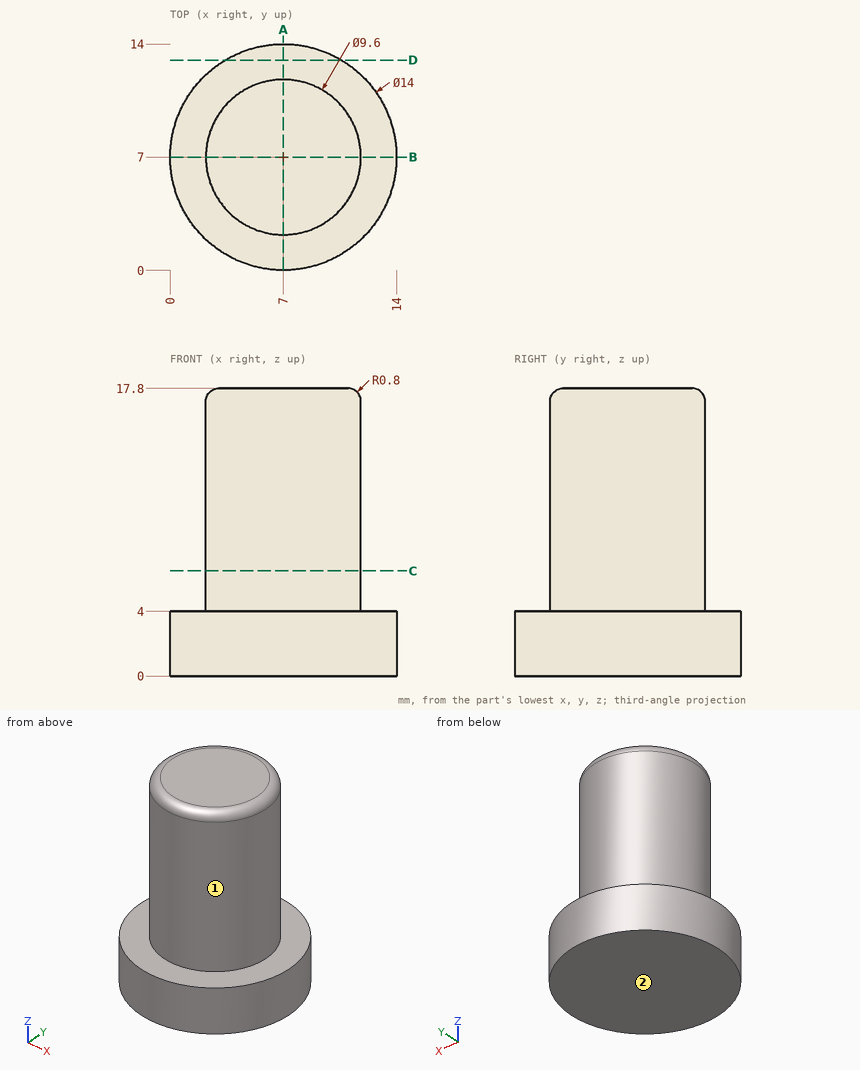
Part print with two shaded views. Sizes in mm from the minimum x, y, z corner. A direction names the side the tool comes from. Give positions to 0.01 mm unless a question says otherwise; leave off trailing zeros. Order: outer loops, then holes, each group sorted by start corner. A loop starts at its lowest first (then second) coordinate and runs counter-clockwise, first axis right, second up.
(1) Tool access for the marked faces 1 and 2: list every direction of +Z, -Z, +X, -X, +Y, -Y with a clear straight run to the whole face (end or side of a thin tool).
(2) Saw through at D-D, the plane y = 13. Give the cut face in (x, z), then the cut area to 3 significant figures.
(3) Saw through at A-A, the plane x = 7. Give the cut face in (y, z).
(4) Flat gauge pins, fed straight in: pin 1 (5 mm diameter, centred on x = 9.5, z = 5.5, fed in from +Y); pin 2 (6 mm diameter, centred on y = 8.5, z = 11.5, fed in from -X); pin 3 (2 mm diameter, centred on x = 7.5, z = 11, fed in from -Y). Where does each tip first touch, or does it go through?
(5) Saw through at C-C, the plane z = 6.5. Give the cut face in (x, y).
(6) Drill centre lines: L1, parallel to Z at x = 10.25, y = 11.5; L2, parallel to Y at x = 7.25, z = 0.75; L3, parallel to X at y = 4.75, z = 10. Where is each one in solid material? Low to high.
Results found:
1. face 1: +Z
1. face 2: -Z, +X, -X, +Y, -Y
2. outline: (3.39, 0) - (10.61, 0) - (10.61, 4) - (3.39, 4) - close
2. area: 28.8 mm2
3. outline: (0, 0) - (14, 0) - (14, 4) - (11.8, 4) - (11.8, 17) arc R0.8 ccw to (11, 17.8) - (3, 17.8) arc R0.8 ccw to (2.2, 17) - (2.2, 4) - (0, 4) - close
4. pin 1: stops at y = 13.98
4. pin 2: stops at x = 2.2
4. pin 3: stops at y = 2.2
5. outline: circle Ø9.6 at (7, 7)
6. L1: z = 0 to 4
6. L2: y = 0 to 14
6. L3: x = 2.76 to 11.24
